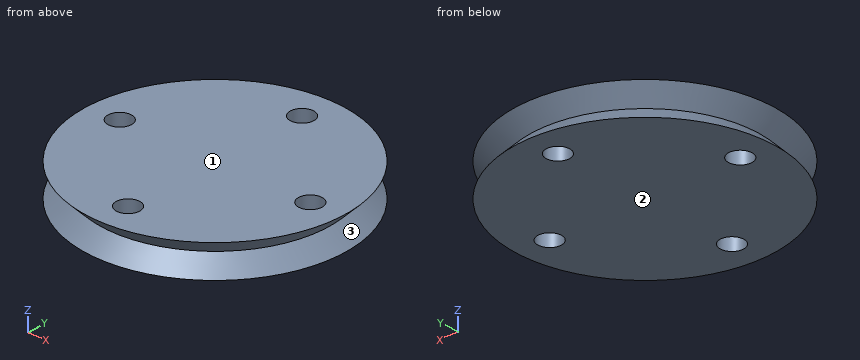
from build123d import *

# Parameters (mm, degrees)
SKETCH1_R           = 8
BOSS_EXTRUDE1_DEPTH = 2
SKETCH2_R           = 0.726422571
CUT_EXTRUDE1_DEPTH  = 2


with BuildPart() as part:
    # Sketch1 → Boss-Extrude1 (new body)
    with BuildSketch(Plane.XY):
        Circle(SKETCH1_R)
    extrude(amount=BOSS_EXTRUDE1_DEPTH)

    # Sketch2 → Cut-Extrude1 (cut)
    with BuildSketch(Plane.XY):
        with Locations((-6, 0)):
            Circle(SKETCH2_R)
        with Locations((0, 6)):
            Circle(SKETCH2_R)
        with Locations((6, 0)):
            Circle(SKETCH2_R)
        with Locations((0, -6)):
            Circle(SKETCH2_R)
    extrude(amount=CUT_EXTRUDE1_DEPTH, mode=Mode.SUBTRACT)

    # Sketch3 → Cut-Revolve1 (revolve, cut)
    with BuildSketch(Plane(origin=(0, 0, 0), x_dir=(0, 0, -1), z_dir=(1, 0, 0))):
        Polygon((-2, 8), (-1, 7), (0, 8), align=None)
    revolve(axis=Axis((0, 0, 3.502327543), (0, 0, -1)), mode=Mode.SUBTRACT)


solid = part.part
Geometry check sheet. Reference: the model listing, model coordinates, mm. Face numbers are marked on the shaded views. Give positions to 0.01 mm unless a question says otherwise; leave off trailing zeros. Loops run counter-clockwise (first coordinate to the right, second up) from the corner with the lowest first, then second, coordinate; pieces in that order, holes last.
(1) Section check D-D on z = 0.25. Record the cut outline in (x, y).
From the geometry:
outline: circle Ø15.5 at (0, 0); hole circle Ø1.45 at (-6, 0); hole circle Ø1.45 at (0, -6); hole circle Ø1.45 at (0, 6); hole circle Ø1.45 at (6, 0)
(2) Depth check by flat-ended pin: pin 1 Ø1.2 at (x, y) = (6, 0) entering from -Z; pin 2 Ø1 at (x, z) = (6, 0.5) entering from +Y. Enter the tip coordinate at first touch or a pass-through.
From the geometry:
pin 1: passes through
pin 2: stops at y = 5.47
(3) Section check B-B on y = -0.5. Count the separate pieces of the cut face and the enclosed holes in it, then the cut area to 3 significant figures.
From the geometry:
separate pieces: 3
enclosed holes: 0
area: 25.7 mm2
(4) Release check for a two-part mould opening along Z. For the marked faces 1, 2 and 3 record: released by +Z, released by -Z, zero draft, split by the parting line, or undercut.
From the geometry:
face 1: released by +Z
face 2: released by -Z
face 3: undercut
(5) Thickness scan on L1, parallel to Y at x = -6, z = 0.8; L2, parallel to X at y = -6.25, z = 1.75; L3, parallel to Y at x = -0.5, z = 1.3. Record the ranges inside material, lowest first.
From the geometry:
L1: y = -3.98 to -0.73, 0.73 to 3.98
L2: x = -4.58 to -0.68, 0.68 to 4.58
L3: y = -7.28 to -6.53, -5.47 to 5.47, 6.53 to 7.28
(6) Section check A-A on z = 1.3. Record the cut outline in (x, y).
From the geometry:
outline: circle Ø14.6 at (0, 0); hole circle Ø1.45 at (-6, 0); hole circle Ø1.45 at (0, -6); hole circle Ø1.45 at (0, 6); hole circle Ø1.45 at (6, 0)
